Answer from the drawing. Dimensions are ordinates in mm from the lowest x, y and z of the part. Round coordinates to 2 decimals unless told otherwise and drop trailing zeros. Loops run counter-clockwise (first coordinate to the right, second up) from the corner with the lowest first, then second, coordinate; pieces in that order, holes last. Notation, with made-up numbers: (47.25, 13.25) - (61.25, 13.25) arc R33 ccw to (61.25, 45.25) - close; hole circle Ø10 at (-21.75, 30). An arc over 180 degrees is marked (long way). Answer as CSV lines item,"result".
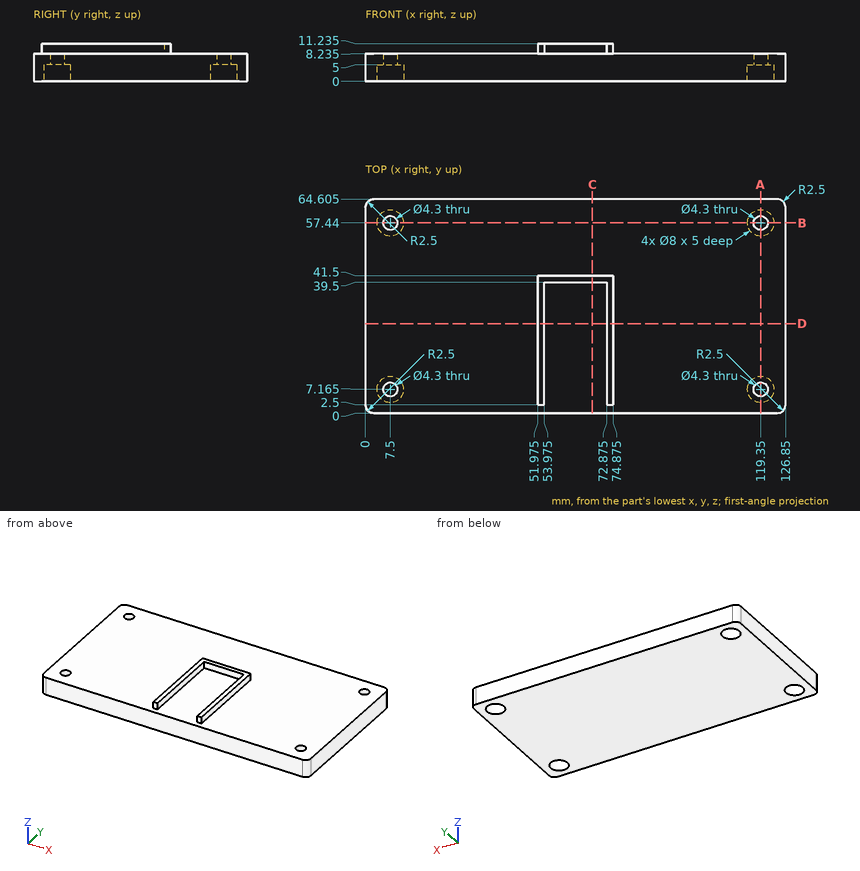
1) A cutting plane is placed at C-C, the plane x = 68.5. Determine the outline of the cut face in (y, z) (3 decimals), plus the area to 3 significant figures.
Entries:
outline,"(0, 0) - (64.605, 0) - (64.605, 8.235) - (41.5, 8.235) - (41.5, 11.235) - (39.5, 11.235) - (39.5, 8.235) - (0, 8.235) - close"
area,"538 mm^2"
2) Find the intervals of material crossed by line 1 (X direction, y = 57.44, z = 5.95); line 2 (Y direction, x = 119.5, z = 7.75) (3 decimals); line 3 (X direction, y = 55, z = 3.25), in increasing order.
Entries:
line 1,"x = 0 to 5.35, 9.65 to 117.2, 121.5 to 126.85"
line 2,"y = 0 to 5.02, 9.31 to 55.295, 59.585 to 64.605"
line 3,"x = 0 to 4.33, 10.67 to 116.18, 122.52 to 126.85"
3) A cutting plane is placed at D-D, the plane y = 27. Determine the outline of the cut face in (x, z) (3 decimals).
Entries:
outline,"(0, 0) - (126.85, 0) - (126.85, 8.235) - (74.875, 8.235) - (74.875, 11.235) - (72.875, 11.235) - (72.875, 8.235) - (53.975, 8.235) - (53.975, 11.235) - (51.975, 11.235) - (51.975, 8.235) - (0, 8.235) - close"
4) A cutting plane is placed at B-B, the plane y = 57.44. Determine the outline of the cut face in (x, z) (3 decimals).
Entries:
outline,"(0, 0) - (3.5, 0) - (3.5, 5) - (5.35, 5) - (5.35, 8.235) - (0, 8.235) - close; (9.65, 5) - (11.5, 5) - (11.5, 0) - (115.35, 0) - (115.35, 5) - (117.2, 5) - (117.2, 8.235) - (9.65, 8.235) - close; (121.5, 5) - (123.35, 5) - (123.35, 0) - (126.85, 0) - (126.85, 8.235) - (121.5, 8.235) - close"
5) Each of these flat-tipped pins is pushed along its axis until it touches: P1, Ø0.9, axis at y = 28, z = 10.5, coming from the -X side (3 decimals); P2, Ø7, axis at x = 119.35, y = 7.165, coming from the -Z side; P3, Ø0.6, axis at x = 73.5, z = 10, coming from the -Y side. Where does it stop, or does it pass through?
Entries:
P1,"stops at x = 51.975"
P2,"stops at z = 5"
P3,"stops at y = 2.5"
6) A cutting plane is placed at A-A, the plane x = 119.35. Determine the outline of the cut face in (y, z) (3 decimals), plus the area to 3 significant figures.
Entries:
outline,"(0, 0) - (3.165, 0) - (3.165, 5) - (5.015, 5) - (5.015, 8.235) - (0, 8.235) - close; (9.315, 5) - (11.165, 5) - (11.165, 0) - (53.44, 0) - (53.44, 5) - (55.29, 5) - (55.29, 8.235) - (9.315, 8.235) - close; (59.59, 5) - (61.44, 5) - (61.44, 0) - (64.605, 0) - (64.605, 8.235) - (59.59, 8.235) - close"
area,"424 mm^2"
